The listing builds one solid part. Answer for the finished solid, in the listing's coordinates (mm). Face numbers are marked on the shaded views. A direction names the side the tool comes from. Give positions to 0.01 mm unless a question says otherwise; leave off trailing zeros. Write each loop counter-clockwise with the first axis right and the second up, starting at its lowest first coordinate (ties: lowest second). Pieces come first, ordered by that corner, then holes. Notation, with made-up numbers: (86, -10.75) - (128, -10.75) arc R13 cw to (128, 7.25) - close; hole circle Ø8 at (12, 9). An arc over 180 degrees is marked (long way). Write each question's results on one line, items separated by ' | '. Start each with the question number.
Q1. Section B-B (y = 0.8) is taken. Determine the outline of the cut face in (x, z).
Q2. For a pull along Z with two mould halves and no side action, classify the marked faces 3, 4, 5 and 6 as pulls with the +Z half, pulls with the -Z half, needs draft (parallel to the pull), parting line crosses it, or undercut.
Q3. Flat-ended cylindrical pins translate along their axes: pin 1 Ø2 at (y, z) = (0.5, -1.5) entering from -X; pin 2 Ø3 at (x, z) = (-2, -8.5) entering from +Y; pin 3 Ø1.5 at (x, y) = (0.5, 3.5) entering from +Z. Find the tip coordinate at first contact, or state that the pin passes through.
Q4. Section D-D (x = 0) is taken. Determine the outline of the cut face in (y, z).
Q5. Section A-A (z = 0) is taken. Determine the outline of the cut face in (x, y), plus the area to 4 significant figures.
Q6. Section C-C (x = -1.5) is taken. Determine the outline of the cut face in (y, z), plus the area to 3 significant figures.
Q7. For the marked faces 1 and 2, determine the directions among +Z, -Z, +X, -X, +Y, -Y from which every point of the face is accessible in a straight line to the end or side of a thin tool.
Q8. Find the intervals of material crossed by probe 1 along X at (y, z) = (1.45, 0); probe 2 along Y at (x, z) = (0.75, -5); probe 3 along Z at (x, y) = (2.25, 3.55), in increasing order.
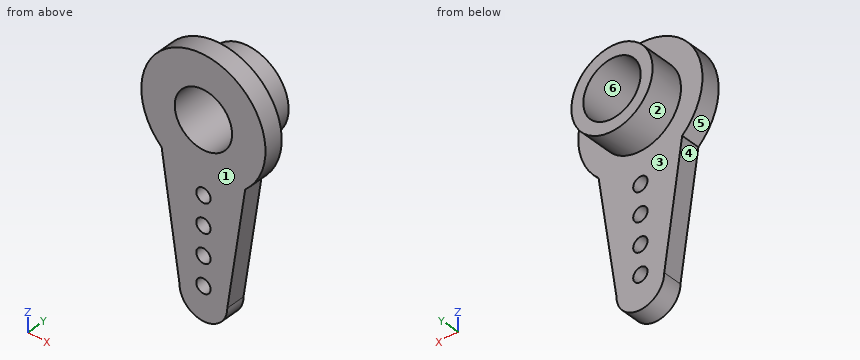
```python
from build123d import *

# Parameters (mm, degrees)
AUFSATZ_LINEAR_AUSTRAGEN1_DEPTH = 2
SKIZZE2_R                       = 4.25
SKIZZE2_R_2                     = 3
AUFSATZ_LINEAR_AUSTRAGEN2_DEPTH = 3.5
SCHNITT_LINEAR_START            = -3.5
SKIZZE3_R                       = 3
SCHNITT_LINEAR_AUSTRAGEN1_DEPTH = 3.5
SKIZZE4_R                       = 0.75
SCHNITT_LINEAR_AUSTRAGEN2_DEPTH = 3.5


with BuildPart() as part:
    # Skizze1 → Aufsatz-Linear austragen1 (new body)
    with BuildSketch(Plane(origin=(0, 0, 0), x_dir=(1, 0, 0), z_dir=(0, 1, 0))):
        with BuildLine():
            Line((-2.5, 17.5), (-4.374965285, 4.807252725))
            ThreePointArc((-4.374965285, 4.807252725), (0, -6.5), (4.374965285, 4.807252725))
            Line((4.374965285, 4.807252725), (2.5, 17.5))
            ThreePointArc((2.5, 17.5), (0, 20), (-2.5, 17.5))
        make_face()
    extrude(amount=AUFSATZ_LINEAR_AUSTRAGEN1_DEPTH)

    # Skizze2 → Aufsatz-Linear austragen2 (add)
    with BuildSketch(Plane(origin=(0, 2, 0), x_dir=(1, 0, 0), z_dir=(0, 1, 0))):
        with Locations(Location((0, 0, 0), (0, 0, 270))):
            Circle(SKIZZE2_R)
        with Locations(Location((0, 0, 0), (0, 0, 270))):
            Circle(SKIZZE2_R_2, mode=Mode.SUBTRACT)
    extrude(amount=AUFSATZ_LINEAR_AUSTRAGEN2_DEPTH)

    # Skizze3 → Schnitt-Linear austragen1 (cut)
    with BuildSketch(Plane(origin=(0, 2, 0), x_dir=(1, 0, 0), z_dir=(0, 1, 0)).offset(SCHNITT_LINEAR_START)):
        with Locations(Location((0, 0, 0), (0, 0, 270))):
            Circle(SKIZZE3_R)
    extrude(amount=SCHNITT_LINEAR_AUSTRAGEN1_DEPTH, mode=Mode.SUBTRACT)

    # Skizze4 → Schnitt-Linear austragen2 (cut)
    with BuildSketch(Plane(origin=(0, 2, 0), x_dir=(1, 0, 0), z_dir=(0, 1, 0))):
        with Locations(Location((0, 7.5, 0), (0, 0, 270))):
            Circle(SKIZZE4_R)
        with Locations(Location((0, 10.5, 0), (0, 0, 270))):
            Circle(SKIZZE4_R)
        with Locations(Location((0, 13.5, 0), (0, 0, 270))):
            Circle(SKIZZE4_R)
        with Locations(Location((0, 16.5, 0), (0, 0, 270))):
            Circle(SKIZZE4_R)
    extrude(amount=-SCHNITT_LINEAR_AUSTRAGEN2_DEPTH, mode=Mode.SUBTRACT)


solid = part.part
```
Answers below:
1) outline: (-4.37, -4.81) - (-2.5, -17.5) arc R2.5 ccw to (2.5, -17.5) - (4.37, -4.81) arc R6.5 ccw (long way) to start; hole circle Ø6 at (0, 0); hole circle Ø1.5 at (0, -16.5); hole circle Ø1.5 at (0, -13.5); hole circle Ø1.5 at (0, -10.5); hole circle Ø1.5 at (0, -7.5)
2) face 3: needs draft | face 4: pulls with the -Z half | face 5: parting line crosses it | face 6: undercut
3) pin 1: stops at x = -6.48 | pin 2: stops at y = 2 | pin 3: stops at z = 4.25
4) outline: (0, -20) - (2, -20) - (2, -17.25) - (0, -17.25) - close; (0, -15.75) - (2, -15.75) - (2, -14.25) - (0, -14.25) - close; (0, -12.75) - (2, -12.75) - (2, -11.25) - (0, -11.25) - close; (0, -9.75) - (2, -9.75) - (2, -8.25) - (0, -8.25) - close; (0, -6.75) - (2, -6.75) - (2, -4.25) - (5.5, -4.25) - (5.5, -3) - (0, -3) - close; (0, 3) - (5.5, 3) - (5.5, 4.25) - (2, 4.25) - (2, 6.5) - (0, 6.5) - close
5) outline: (-6.5, 0) - (-3, 0) - (-3, 5.5) - (-4.25, 5.5) - (-4.25, 2) - (-6.5, 2) - close; (3, 0) - (6.5, 0) - (6.5, 2) - (4.25, 2) - (4.25, 5.5) - (3, 5.5) - close | area: 22.75 mm2
6) outline: (0, -19.5) - (2, -19.5) - (2, -3.98) - (5.5, -3.98) - (5.5, -2.6) - (0, -2.6) - close; (0, 2.6) - (5.5, 2.6) - (5.5, 3.98) - (2, 3.98) - (2, 6.32) - (0, 6.32) - close | area: 50.9 mm2
7) face 1: +Z, -Z, +X, -X, -Y | face 2: +Y
8) probe 1: x = -6.5 to -3, 3 to 6.5 | probe 2: y = 0 to 2 | probe 3: z = -3.61 to -1.98, 1.98 to 3.61
